Work out the finished part from the listing and answer in its coordinate system (mm). A direction names the side the tool comes from. Give positions to 0.01 mm unless a question says otherwise; leave off trailing zeros. Loops run counter-clockwise (first coordinate to the right, second up) from the corner with the lowest first, then second, coordinate; pieces in that order, holes last.
```python
from build123d import *

# Parameters (mm, degrees)
SKETCH1_R           = 4.15
SKETCH1_R_2         = 9.6
BOSS_EXTRUDE1_DEPTH = 2


with BuildPart() as part:
    # Sketch1 → Boss-Extrude1 (new body)
    with BuildSketch(Plane.XY):
        with BuildLine():
            Line((-14.85, 29), (-14.85, 26.25))
            ThreePointArc((-14.85, 26.25), (-15.655456352, 24.305456352), (-17.6, 23.5))
            Line((-17.6, 23.5), (-20, 23.5))
            Line((-20, 23.5), (-20, -23.5))
            Line((-20, -23.5), (-17.6, -23.5))
            ThreePointArc((-17.6, -23.5), (-15.655456352, -24.305456352), (-14.85, -26.25))
            Line((-14.85, -26.25), (-14.85, -29))
            Line((-14.85, -29), (14.85, -29))
            Line((14.85, -29), (14.85, -26.25))
            ThreePointArc((14.85, -26.25), (15.655456352, -24.305456352), (17.6, -23.5))
            Line((17.6, -23.5), (20, -23.5))
            Line((20, -23.5), (20, 23.5))
            Line((20, 23.5), (17.6, 23.5))
            ThreePointArc((17.6, 23.5), (15.655456352, 24.305456352), (14.85, 26.25))
            Line((14.85, 26.25), (14.85, 29))
            Line((14.85, 29), (-14.85, 29))
        make_face()
        with Locations((-13.75, -19.7)):
            Circle(SKETCH1_R, mode=Mode.SUBTRACT)
        with Locations((-5.725, -6.1)):
            Circle(SKETCH1_R, mode=Mode.SUBTRACT)
        with BuildLine():
            ThreePointArc((16.186, -16.278610808), (17.171389192, -22.136), (11.314, -23.121389192))
            Line((11.314, -23.121389192), (7.240917629, -20.221389192))
            ThreePointArc((7.240917629, -20.221389192), (6.255528438, -14.364), (12.112917629, -13.378610808))
            Line((12.112917629, -13.378610808), (16.186, -16.278610808))
        make_face(mode=Mode.SUBTRACT)
        with Locations((5.725, -6.1)):
            Circle(SKETCH1_R, mode=Mode.SUBTRACT)
        with Locations((0, 8.65)):
            Circle(SKETCH1_R_2, mode=Mode.SUBTRACT)
        with Locations((-13.75, 20.15)):
            Circle(SKETCH1_R, mode=Mode.SUBTRACT)
        with Locations((13.75, 20.15)):
            Circle(SKETCH1_R, mode=Mode.SUBTRACT)
    extrude(amount=BOSS_EXTRUDE1_DEPTH)


solid = part.part
```
Q1. Section A-A on x = 0 is taken. Give the vertices of the cut face in (y, z), plus the area to 3 significant figures.
Q2. Section D-D on y = 8.65 is taken. Give the vertices of the cut face in (x, z), plus the area to 3 significant figures.
Q3. Determine the mould class of faces 6 (the face through (-9.018, -8.625, 0.986)), 7 (the face through (20, 0, 1)), 8 (the face through (0, -29, 1)), 9 (the face through (14.12, -14.81, 0.99)) for opening direction Y: +Y half, -Y half, draft (parallel to the pull), parting line (faces both ways), or undercut.
Q4. Section C-C on z = 0.3 is taken. Give the vertices of the cut face in (x, y) (3 decimals), plus the area to 3 significant figures.
Q5. Which of the six approach directions +Z, -Z, +X, -X, +Y, -Y give full straight-line access (tool end or side, diameter ignored) to faces 1 (the face through (19, 23.5, 1)), 2 (the face through (9.306, -21.692, 0.986)), 3 (the face through (-14.85, -28, 1)), 4 (the face through (-14.85, 28, 1)), 5 (the face through (19, -23.5, 1))?
Q6. Consider line 1 along Y through (x, z) = (0, 1.6); line 2 along X through (y, z) = (-18.5, 0.3); line 3 along Y through (x, z) = (-10.5, 0.9). Determine where each line is inside the solid, lowest interval first.
Q7. Section B-B on y = 20.15 is taken. Give the vertices of the cut face in (x, z).
Q8. Given pin 1 (0.6 mm diameter, centred on x = -18.5, z = 1.5, fed in from +Y), flat-ended and moving along its own axis, determine where the tip first touches the part or whether it passes through.
Check result:
1. outline: (-29, 0) - (-0.95, 0) - (-0.95, 2) - (-29, 2) - close; (18.25, 0) - (29, 0) - (29, 2) - (18.25, 2) - close
1. area: 77.6 mm2
2. outline: (-20, 0) - (-9.6, 0) - (-9.6, 2) - (-20, 2) - close; (9.6, 0) - (20, 0) - (20, 2) - (9.6, 2) - close
2. area: 41.6 mm2
3. face 6: undercut
3. face 7: draft
3. face 8: -Y half
3. face 9: undercut
4. outline: (-20, -23.5) - (-17.6, -23.5) arc R2.75 cw to (-14.85, -26.25) - (-14.85, -29) - (14.85, -29) - (14.85, -26.25) arc R2.75 cw to (17.6, -23.5) - (20, -23.5) - (20, 23.5) - (17.6, 23.5) arc R2.75 cw to (14.85, 26.25) - (14.85, 29) - (-14.85, 29) - (-14.85, 26.25) arc R2.75 cw to (-17.6, 23.5) - (-20, 23.5) - close; hole circle Ø8.3 at (-13.75, -19.7); hole circle Ø8.3 at (-13.75, 20.15); hole circle Ø8.3 at (-5.725, -6.1); hole circle Ø19.2 at (0, 8.65); hole circle Ø8.3 at (5.725, -6.1); hole (7.241, -20.221) - (11.314, -23.121) arc R4.2 ccw to (16.186, -16.279) - (12.113, -13.379) arc R4.2 ccw to start; hole circle Ø8.3 at (13.75, 20.15)
4. area: 1,560 mm2
5. face 1: +Z, -Z, +X, +Y
5. face 2: +Z, -Z
5. face 3: +Z, -Z, -X, -Y
5. face 4: +Z, -Z, -X, +Y
5. face 5: +Z, -Z, +X, -Y
6. line 1: y = -29 to -0.95, 18.25 to 29
6. line 2: x = -20 to -17.72, -9.78 to 5.84, 17.77 to 20
6. line 3: y = -29 to -22.28, -17.12 to 17.57, 22.73 to 29
7. outline: (-20, 0) - (-17.9, 0) - (-17.9, 2) - (-20, 2) - close; (-9.6, 0) - (9.6, 0) - (9.6, 2) - (-9.6, 2) - close; (17.9, 0) - (20, 0) - (20, 2) - (17.9, 2) - close
8. pin 1: stops at y = 23.5
